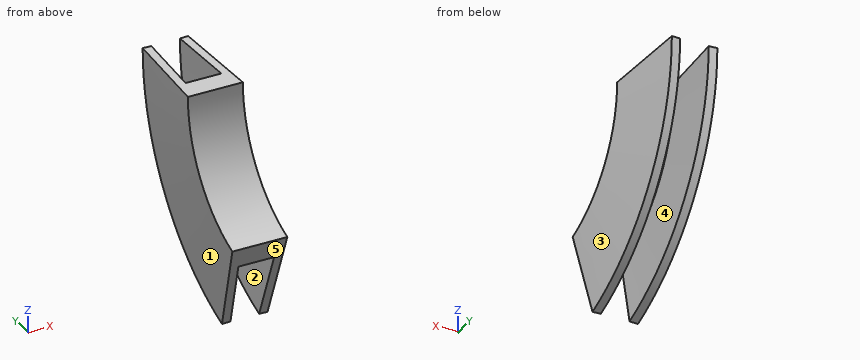
```python
from build123d import *


with BuildPart() as part:
    # Sweep1: sweep along a path in Sketch3
    with BuildLine(Plane(origin=(0, 0, 0), x_dir=(0, 0, -1), z_dir=(1, 0, 0))) as sweep1_path:
        ThreePointArc((0, 0), (7.5, -2.45109762), (12.105002811, -8.858267717))
    # Sketch1 → Sweep1 (sweep)
    with BuildSketch(Plane.XY):
        Polygon((-2.019073099, 6.379558093), (-2.43857571, -2), (2.43857571, -2), (2.019073099, 6.379558093), (1.27, 6.342057533), (1.5875, 0), (-1.5875, 0), (-1.27, 6.342057533), align=None)
    sweep(path=sweep1_path.line)


solid = part.part
```
Check sheet for the modelled part. Datum: model origin and axes. Units: mm. Face numbers are marked on the shaded views. A direction names the side the tool comes from. Give positions to 0.01 mm unless a question says otherwise; leave off trailing zeros. Order: outer loops, then holes, each group sorted by start corner. A loop starts at its lowest first (then second) coordinate and runs counter-clockwise, first axis right, second up. Notation, with made-up numbers: M 73.5,78 L 109.5,78 A29 ccw 109.5,105 Z; hole C 27,39.25 d8. An arc over 180 degrees is marked long. Answer in a Markdown table with one row per item.
1) Access from +Z, -Z, +X, -X, +Y, -Y to the whole of each face (thin tool, end or side, straight path). Record for the marked faces 1 and 2.
Filled sheet:
| item | result |
|---|---|
| face 1 | -Z, -X, +Y |
| face 2 | none |
2) Gauge pin test, flat ends, axial feed: P1, Ø1, axis at x = -0.5, y = -4, coming from the -Z side; P2, Ø2, axis at x = 0, y = -4, coming from the +Z side. Record the tip position at first contact, or that the pin passes through.
Filled sheet:
| item | result |
|---|---|
| P1 | stops at z = -9.7 |
| P2 | stops at z = -4.52 |
3) Thickness scan on L1, parallel to X at y = 2.5, z = -5; L2, parallel to X at y = 1.5, z = -11.25; L3, parallel to Y at x = 0.4, z = -4.5. Record the ranges inside material, lowest first. Write a range as [from, to].
Filled sheet:
| item | result |
|---|---|
| L1 | x = [-2.17, -1.42], [1.42, 2.17] |
| L2 | x = [-2.07, -1.32], [1.32, 2.07] |
| L3 | y = [-2.99, -0.82] |
4) Release check for a two-part mould opening along X. For the marked faces 3, 4 and 5 record: +X half, -X half, draft (parallel to the pull), parting line (faces both ways), or undercut.
Filled sheet:
| item | result |
|---|---|
| face 3 | +X half |
| face 4 | undercut |
| face 5 | draft |
5) Cross-section at A-A, the plane x = 0.15. Enter the section's corners in (y, z) (3 decimals), plus the area to 3 significant figures.
Filled sheet:
| item | result |
|---|---|
| outline | M -9.463,-10.199 L -8.858,-12.105 A12.7 ccw 0,0 L -2,0 A10.7 cw Z |
| area | 29.6 mm2 |
